Input: part model. Units: mm. Frame: model coordinates. Face numbers are marked on the shaded views. A direction names the side the tool comes from. Coordinates: 2 decimals unless noted, no trailing zeros. Loops run counter-clockwise (first coordinate to the right, second up) from the corner with the lowest first, then second, coordinate; pieces in that order, holes last.
(1) Section A-A, the plane y = 0. Return loops of the section in (x, z) (3 decimals), then the cut area to 3 significant figures.
(2) Section C-C, the plane z = 3. Return loops of the section in (x, y).
(3) Line query: L1, parallel to Z at x = 6, y = -13; L2, parallel to Y at x = 17, z = 19; L3, parallel to Z at x = -16.5, y = 6. Output: solid intervals per line, ascending.
(4) Contact query for flat-ended pins moving along their axis: P1, Ø10, axis at y = -15, z = -2.5, coming from the -X side; P2, Ø1.5, axis at x = 13, y = 14, coming from the +Z side; P3, Ø1, axis at x = -11.5, y = -8, coming from the -Z side. Output: stop coordinate, or through.
(5) Set-up query: the marked faces 1 and 2. Return all of +Z, -Z, +X, -X, +Y, -Y with unobstructed straight access to the full face (end or side cutting, diameter ignored); none if empty.
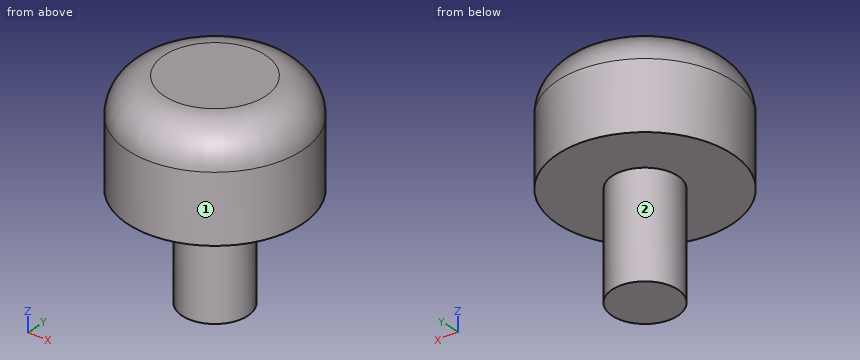
```python
from build123d import *

# Parameters (mm, degrees)
F0_R     = 23.9
F1_DEPTH = 28.5
F2_R     = 8.98
F3_DEPTH = 28.575
F4_R     = 10


# Not quite as in the source:
# - a length typed as a fraction of an inch, garbled in the dataset ("3 / 203.2 mm" for 3/8 in), is restored


with BuildPart() as f1:
    # F0 (on Top) → F1 (new body)
    with BuildSketch(Plane.XY):
        Circle(F0_R)
    extrude(amount=F1_DEPTH)

    # F2 (on face) → F3 (join)
    with BuildSketch(Plane(origin=(0, 0, 0), x_dir=(1, 0, 0), z_dir=(0, 0, -1))):
        Circle(F2_R)
    extrude(amount=F3_DEPTH)

    # F4
    f4_edges = [f1.edges().sort_by_distance(p)[0] for p in [
        (-23.9, 0, 28.5),
    ]]
    fillet(f4_edges, radius=F4_R)


solid = f1.part
```
Report:
1. outline: (-23.9, 0) - (-8.98, 0) - (-8.98, -28.575) - (8.98, -28.575) - (8.98, 0) - (23.9, 0) - (23.9, 18.5) arc R10 ccw to (13.9, 28.5) - (-13.9, 28.5) arc R10 ccw to (-23.9, 18.5) - close
1. area: 1,830 mm2
2. outline: circle Ø47.8 at (0, 0)
3. L1: z = 0 to 28.49
3. L2: y = -16.78 to 16.78
3. L3: z = 0 to 27.81
4. P1: stops at x = -21.39
4. P2: stops at z = 27.45
4. P3: stops at z = 0
5. face 1: +Z, -Z
5. face 2: -Z
